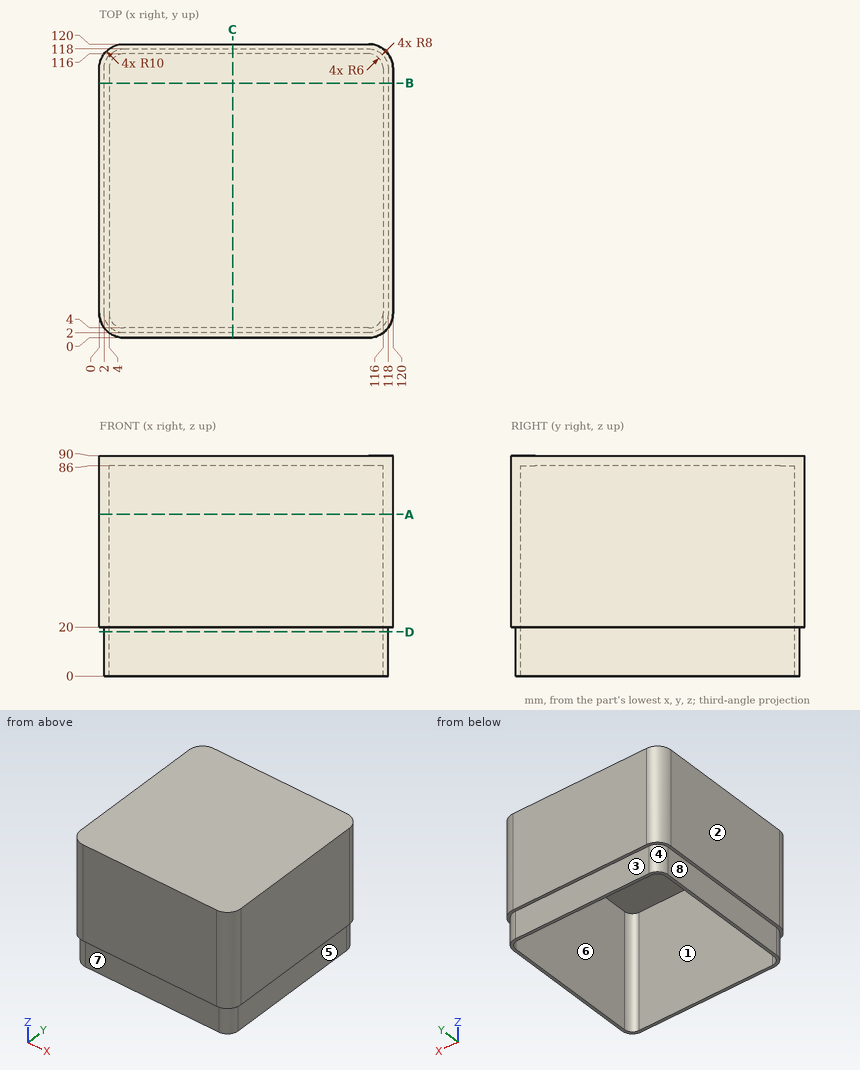
Answer from the drawing. Dimensions are ordinates in mm from the lowest x, y and z of the part. A direction names the side the tool comes from. Give positions to 0.01 mm unless a question says otherwise; leave off trailing zeros. Order: outer loops, then holes, each group sorted by start corner. A loop starts at its lowest first (then second) coordinate and runs counter-clockwise, first axis right, second up.
(1) For a pull along Y with two mould halves and no side action, classify the marked faces 1, 2 and 3 as released by +Y, released by -Y, zero draft, split by the parting line, or undercut.
(2) Find section D-D (z = 18). Give the vertices of the cut face in (x, y), plus the area to 3 significant figures.
(3) Find section B-B (y = 104). Give the vertices of the cut face in (x, z).
(4) Straight lines are drawn through the part: L1, parallel to Y at x = 33.5, z = 56; L2, parallel to Z at x = 107.5, y = 64. For each, find the intervals that lie inside material, in ascending order.
(5) Given pin 1 (4 mm diameter, centred on x = 96.5, y = 91, fed in from -Z); pin 2 (10 mm diameter, centred on y = 72.5, z = 9.5, fed in from -X); pin 3 (10 mm diameter, centred on x = 50.5, z = 11, fed in from -Y), each flat-ended and moving along its own axis, determine where each tip first touches the part or whether it passes through.
(6) For the marked faces 4, 5, 6, 7 and 8, determine the directions among +Z, -Z, +X, -X, +Y, -Y from which every point of the face is accessible in a straight line to the end or side of a thin tool.
(7) Find section A-A (z = 66). Give the vertices of the cut face in (x, y).
Result sheet:
1. face 1: undercut
1. face 2: zero draft
1. face 3: released by +Y
2. outline: (2, 10) arc R8 ccw to (10, 2) - (110, 2) arc R8 ccw to (118, 10) - (118, 110) arc R8 ccw to (110, 118) - (10, 118) arc R8 ccw to (2, 110) - close; hole (4, 10) arc R6 ccw to (10, 4) - (110, 4) arc R6 ccw to (116, 10) - (116, 110) arc R6 ccw to (110, 116) - (10, 116) arc R6 ccw to (4, 110) - close
2. area: 888 mm2
3. outline: (0, 20) - (2, 20) - (2, 0) - (4, 0) - (4, 86) - (116, 86) - (116, 0) - (118, 0) - (118, 20) - (120, 20) - (120, 90) - (0, 90) - close
4. L1: y = 0 to 4, 116 to 120
4. L2: z = 86 to 90
5. pin 1: stops at z = 86
5. pin 2: stops at x = 2
5. pin 3: stops at y = 2
6. face 4: -Z, -X, +Y
6. face 5: -Z, +X, +Y, -Y
6. face 6: -Z
6. face 7: -Z, +X, -X, -Y
6. face 8: -Z, -X, +Y, -Y
7. outline: (0, 10) arc R10 ccw to (10, 0) - (110, 0) arc R10 ccw to (120, 10) - (120, 110) arc R10 ccw to (110, 120) - (10, 120) arc R10 ccw to (0, 110) - close; hole (4, 10) arc R6 ccw to (10, 4) - (110, 4) arc R6 ccw to (116, 10) - (116, 110) arc R6 ccw to (110, 116) - (10, 116) arc R6 ccw to (4, 110) - close
